Design review of the part shown in the three views and the two pictorial views. Dimensions are in mm from the part's minimum x, y and z. A direction names the side the tool comes from. Round coordinates to 2 decimals unless told otherwise and drop trailing zeros. Loops run counter-clockwise (first coordinate to the right, second up) from the corner with the lowest first, then second, coordinate; pieces in that order, holes last. Notation, with made-up numbers: M 15.25,51 L 41.25,51 A26 cw 41.25,67 Z; hole C 31.25,72.25 d11. An arc over 180 degrees is marked long. Answer in a Markdown table with one row per item. Add a question column.
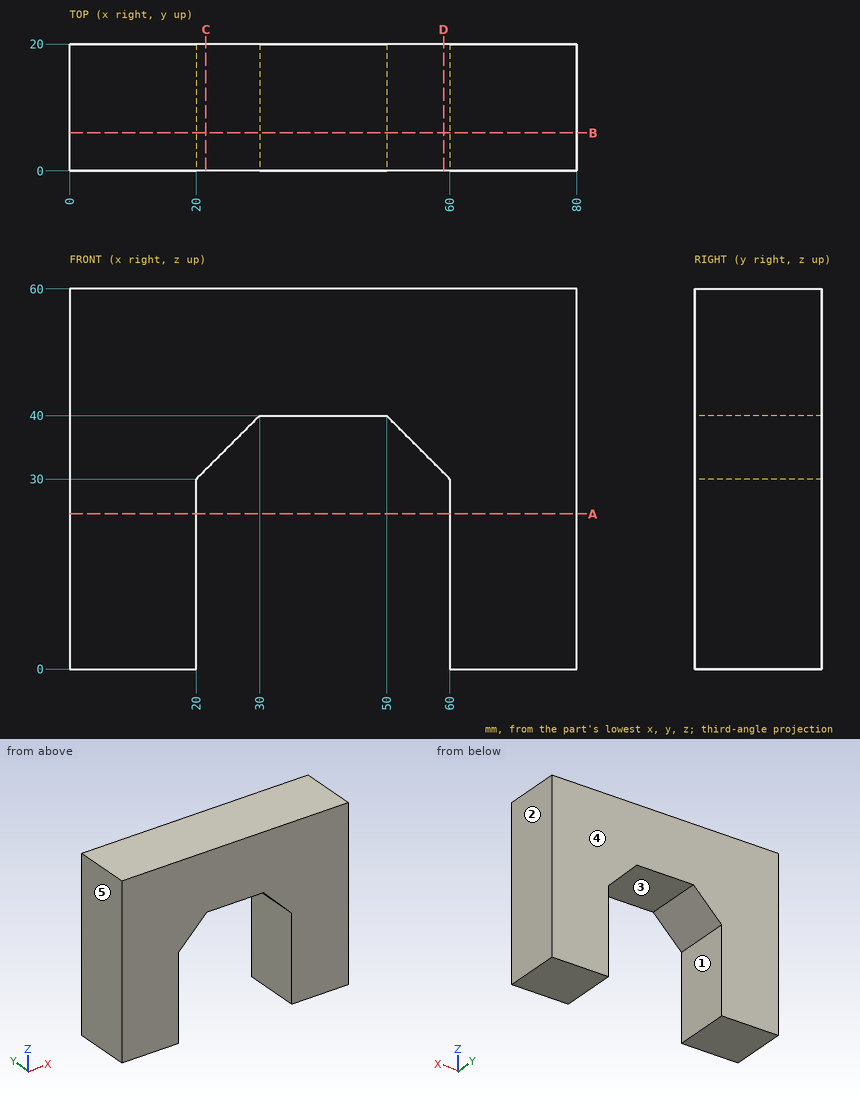
1. Mouldability with a two-part tool opening along X and no side actions: class the marked faces 3, 4 and 5 as released by +X, released by -X, zero draft, split by the parting line, or undercut.
2. Machinability: for the marked faces 1 and 2, which of the approach directions +Z, -Z, +X, -X, +Y, -Y give a long, thin tool a straight path to every point of the face, cutting with its end or side? Answer none if there is none.
3. Take a section at B-B, the plane y = 6. State the section outline as (x, z) points, and give its area (3 significant figures).
4. To check wall thickness, follow probe 1 along X at (y, z) = (4, 19); probe 2 along Z at (x, y) = (48.5, 3); probe 3 along X at (y, z) = (17.5, 30.5). State the ranges of each line that lie inside material, in increasing order.
5. Take a section at C-C, the plane x = 21.5. State the section outline as (y, z) points.
6. Take a section at A-A, the plane z = 24.5. State the section outline as (x, y) points, and give its area (3 significant figures).
7. Take a section at D-D, the plane x = 59. State the section outline as (y, z) points, and give its area (3 significant figures).
Check sheet entries:
| question | item | result |
|---|---|---|
| 1 | face 3 | undercut |
| 1 | face 4 | zero draft |
| 1 | face 5 | released by -X |
| 2 | face 1 | -Z, +Y, -Y |
| 2 | face 2 | +Z, -Z, +X, +Y, -Y |
| 3 | outline | M 0,0 L 20,0 L 20,30 L 30,40 L 50,40 L 60,30 L 60,0 L 80,0 L 80,60 L 0,60 Z |
| 3 | area | 3,300 mm^2 |
| 4 | probe 1 | x = 0 to 20, 60 to 80 |
| 4 | probe 2 | z = 40 to 60 |
| 4 | probe 3 | x = 0 to 20.5, 59.5 to 80 |
| 5 | outline | M 0,31.5 L 20,31.5 L 20,60 L 0,60 Z |
| 6 | outline | M 0,0 L 20,0 L 20,20 L 0,20 Z; M 60,0 L 80,0 L 80,20 L 60,20 Z |
| 6 | area | 800 mm^2 |
| 7 | outline | M 0,31 L 20,31 L 20,60 L 0,60 Z |
| 7 | area | 580 mm^2 |
